The figure shows three views and two pictorial views of one solid part (mm, origin at its lowest corner). Answer the questions. Give positions to 0.01 mm unless a question says otherwise; leave off trailing zeros. Write each loop counter-clockwise with the first axis right and the second up, starting at its lowest first coordinate (ties: lowest second). Pieces come first, ordered by that corner, then holes. Notation, with made-up numbers: (0.5, 8.25) -> (22.5, 8.25) arc R27 ccw to (22.5, 36.25) -> close; hole circle Ø5 at (42.25, 37). An arc over 180 degrees is marked (long way). Use a Markdown table: item, result.
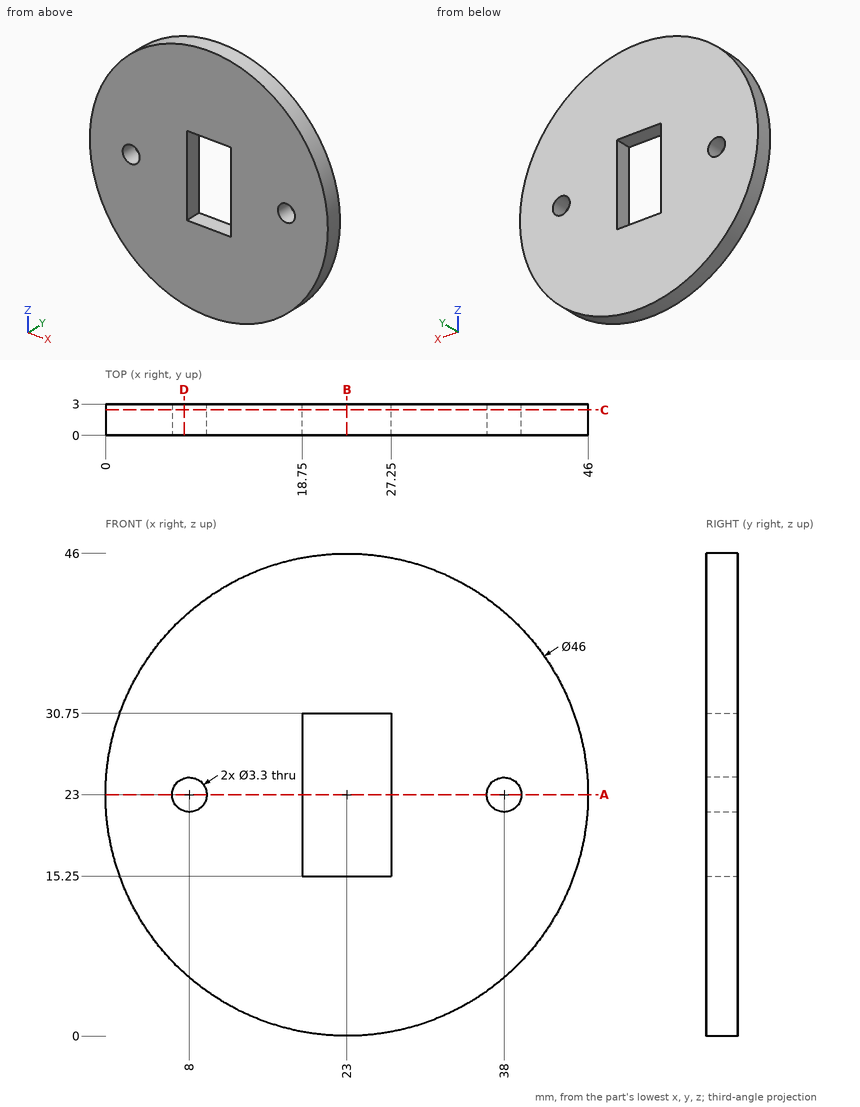
Item 1: A cutting plane is placed at B-B (x = 23). Give the vertices of the cut face in (y, z), then the cut area to 3 significant figures.
Return value:
| item | result |
|---|---|
| outline | (0, 0) -> (3, 0) -> (3, 15.25) -> (0, 15.25) -> close; (0, 30.75) -> (3, 30.75) -> (3, 46) -> (0, 46) -> close |
| area | 91.5 mm^2 |
Item 2: Straight lines are drawn through the part: line 1 along X through (y, z) = (0.65, 23); line 2 along Z through (x, y) = (38, 0.75); line 3 along Z through (x, y) = (37, 2.1). For each, find the intervals that lie inside material, in ascending order. Write a range as [from, to].
Return value:
| item | result |
|---|---|
| line 1 | [0, 6.35], [9.65, 18.75], [27.25, 36.35], [39.65, 46] |
| line 2 | [5.56, 21.35], [24.65, 40.44] |
| line 3 | [4.75, 21.69], [24.31, 41.25] |
Item 3: A cutting plane is placed at D-D (x = 7.5). Give the vertices of the cut face in (y, z).
Return value:
| item | result |
|---|---|
| outline | (0, 6.01) -> (3, 6.01) -> (3, 21.43) -> (0, 21.43) -> close; (0, 24.57) -> (3, 24.57) -> (3, 39.99) -> (0, 39.99) -> close |
Item 4: A cutting plane is placed at A-A (z = 23). Give the vertices of the cut face in (x, y), then the cut area to 3 significant figures.
Return value:
| item | result |
|---|---|
| outline | (0, 0) -> (6.35, 0) -> (6.35, 3) -> (0, 3) -> close; (9.65, 0) -> (18.75, 0) -> (18.75, 3) -> (9.65, 3) -> close; (27.25, 0) -> (36.35, 0) -> (36.35, 3) -> (27.25, 3) -> close; (39.65, 0) -> (46, 0) -> (46, 3) -> (39.65, 3) -> close |
| area | 92.7 mm^2 |
Item 5: A cutting plane is placed at C-C (y = 2.45). Give the vertices of the cut face in (x, z), then the cut area to 3 significant figures.
Return value:
| item | result |
|---|---|
| outline | circle Ø46 at (23, 23); hole circle Ø3.3 at (8, 23); hole (18.75, 15.25) -> (27.25, 15.25) -> (27.25, 30.75) -> (18.75, 30.75) -> close; hole circle Ø3.3 at (38, 23) |
| area | 1,510 mm^2 |
Item 6: Each of these flat-tipped pins is pushed along its axis until it touches: P1, Ø0.9, axis at y = 1, z = 21.5, coming from the +X side; P2, Ø1.5, axis at y = 1.5, z = 26, coming from the -X side. Where does it stop, or does it pass through?
Return value:
| item | result |
|---|---|
| P1 | x = 45.98 |
| P2 | x = 0.11 |
